Could you check a few things on this model? Use its own coordinates, in mm. Face numbers are marked on the shaded views. A direction names the side the tool comes from. Give positions to 0.01 mm unless a question says otherwise; leave off trailing zeros. Order: outer loops, then holes, each group sorted by start corner. A loop starts at its lowest first (then second) coordinate and runs counter-clockwise, first axis right, second up. Notation, with made-up numbers: M -19,42 L -12,42 A27 cw -12,69 Z; hole C -4,12.5 d7. An arc over 180 degrees is marked long. Answer in a Markdown table with one row per item. Add a question column.
```python
from build123d import *

# Parameters (mm, degrees)
SKETCH1_R                = 21
BOSS_EXTRUDE1_DEPTH      = 35
BOSS_EXTRUDE2_DEPTH      = 100
BOSS_EXTRUDE2_DEPTH_BACK = 18
CUT_EXTRUDE2_DEPTH       = 15
SKETCH7_W                = 9
SKETCH7_H                = 30
CUT_EXTRUDE3_DEPTH       = 7
SKETCH8_R                = 1.55
CUT_EXTRUDE4_DEPTH       = 7
SKETCH9_R                = 16.75
CUT_EXTRUDE5_DEPTH       = 20
CUT_EXTRUDE6_DEPTH       = 20
SKETCH11_R               = 1.65
CUT_EXTRUDE9_DEPTH       = 25
SKETCH12_R               = 16.75
CUT_EXTRUDE8_DEPTH       = 10
CUT_EXTRUDE8_DEPTH_BACK  = 25
CUT_EXTRUDE10_DEPTH      = 20
SKETCH15_W               = 65
SKETCH15_H               = 20
BOSS_EXTRUDE3_DEPTH      = 24
SKETCH16_W               = 13
SKETCH16_H               = 16
CUT_EXTRUDE11_DEPTH      = 65


with BuildPart() as part:
    # Sketch1 → Boss-Extrude1 (new body)
    with BuildSketch(Plane(origin=(0, 0, 0), x_dir=(0, 0, -1), z_dir=(1, 0, 0))):
        Circle(SKETCH1_R)
    extrude(amount=BOSS_EXTRUDE1_DEPTH)

    # Sketch4 → Boss-Extrude2 (add, two sides)
    with BuildSketch(Plane.XY) as boss_extrude2_sk:
        with BuildLine():
            Line((35, 21), (35, -21))
            ThreePointArc((35, -21), (56, 0), (35, 21))
        make_face()
    extrude(amount=BOSS_EXTRUDE2_DEPTH)
    extrude(boss_extrude2_sk.sketch, amount=-BOSS_EXTRUDE2_DEPTH_BACK)

    # Sketch5 → Cut-Extrude2 (cut)
    with BuildSketch(Plane.XY.offset(100)):
        with BuildLine():
            Line((45, -18.466185313), (45, 18.466185313))
            ThreePointArc((45, 18.466185313), (56, 0), (45, -18.466185313))
        make_face()
    extrude(amount=-CUT_EXTRUDE2_DEPTH, mode=Mode.SUBTRACT)

    # Sketch7 → Cut-Extrude3 (cut)
    with BuildSketch(Plane.ZY.offset(-35)):
        with Locations((92.5, 0)):
            Rectangle(SKETCH7_W, SKETCH7_H)
    extrude(amount=-CUT_EXTRUDE3_DEPTH, mode=Mode.SUBTRACT)

    # Sketch8 → Cut-Extrude4 (cut)
    with BuildSketch(Plane.ZY.offset(-42)):
        with Locations((92.5, 6.5)):
            Circle(SKETCH8_R)
        with Locations((92.5, 0)):
            Circle(SKETCH8_R)
        with Locations((92.5, -6.5)):
            Circle(SKETCH8_R)
    extrude(amount=-CUT_EXTRUDE4_DEPTH, mode=Mode.SUBTRACT)

    # Sketch9 → Cut-Extrude5 (cut)
    with BuildSketch(Plane.ZY):
        Circle(SKETCH9_R)
    extrude(amount=-CUT_EXTRUDE5_DEPTH, mode=Mode.SUBTRACT)

    # Sketch10 → Cut-Extrude6 (cut)
    with BuildSketch(Plane.ZY):
        with BuildLine():
            Line((15.02133973, 14.675127009), (12.173811363, 11.504817117))
            ThreePointArc((12.173811363, 11.504817117), (16.743318767, -0.473050368), (11.504817117, -12.173811363))
            Line((11.504817117, -12.173811363), (14.675127009, -15.02133973))
            ThreePointArc((14.675127009, -15.02133973), (20.998573008, -0.244809363), (15.02133973, 14.675127009))
        make_face()
    extrude(amount=-CUT_EXTRUDE6_DEPTH, mode=Mode.SUBTRACT)

    # Sketch11 → Cut-Extrude9 (cut)
    with BuildSketch(Plane.ZY.offset(-20)):
        with Locations((-8.485281374, 8.485281374)):
            Circle(SKETCH11_R)
        with Locations((8.485281374, 8.485281374)):
            Circle(SKETCH11_R)
        with Locations((8.485281374, -8.485281374)):
            Circle(SKETCH11_R)
        with Locations((-8.485281374, -8.485281374)):
            Circle(SKETCH11_R)
    extrude(amount=-CUT_EXTRUDE9_DEPTH, mode=Mode.SUBTRACT)

    # Sketch12 → Cut-Extrude8 (cut, two sides)
    with BuildSketch(Plane.ZY.offset(-35)) as cut_extrude8_sk:
        Circle(SKETCH12_R)
    extrude(amount=CUT_EXTRUDE8_DEPTH, mode=Mode.SUBTRACT)
    extrude(cut_extrude8_sk.sketch, amount=-CUT_EXTRUDE8_DEPTH_BACK, mode=Mode.SUBTRACT)

    # Sketch14 → Cut-Extrude10 (cut)
    with BuildSketch(Plane.ZY):
        with BuildLine():
            Line((-14.710965935, 14.986243067), (-11.829145313, 11.858913153))
            ThreePointArc((-11.829145313, 11.858913153), (-16.749986774, 0.021049042), (-11.858913153, -11.829145313))
            Line((-11.858913153, -11.829145313), (-14.986243067, -14.710965935))
            ThreePointArc((-14.986243067, -14.710965935), (-20.999097868, 0.194650327), (-14.710965935, 14.986243067))
        make_face()
    extrude(amount=-CUT_EXTRUDE10_DEPTH, mode=Mode.SUBTRACT)

    # Sketch15 → Boss-Extrude3 (add)
    with BuildSketch(Plane.ZY.offset(-35)):
        with Locations((52.5, 0)):
            Rectangle(SKETCH15_W, SKETCH15_H)
    extrude(amount=BOSS_EXTRUDE3_DEPTH)

    # Sketch16 → Cut-Extrude11 (cut)
    with BuildSketch(Plane.XY.offset(85)):
        with Locations((20.5, 0)):
            Rectangle(SKETCH16_W, SKETCH16_H)
    extrude(amount=-CUT_EXTRUDE11_DEPTH, mode=Mode.SUBTRACT)


solid = part.part
```
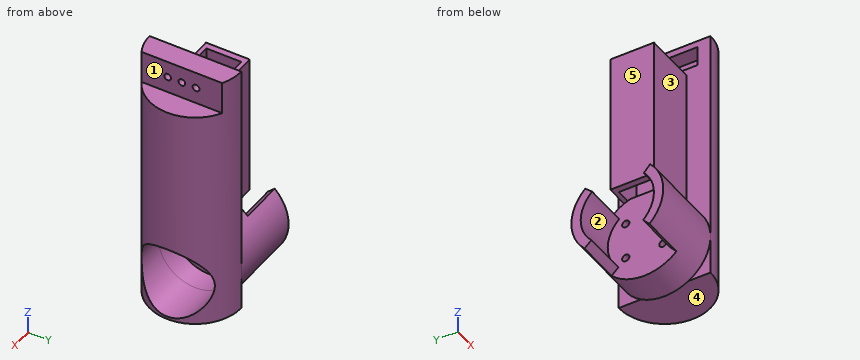
1. Suppose I cut it at D-D on x = 18.5. List the corners of the cut face in (y, z) for me.
2. If I drill on line 1 along Y through (x, z) = (31, 0); line 2 along X through (y, z) = (1, 57); line 3 along Z through (x, y) = (37.5, -4.5), over which ranges is the centre line in solid material (lowest first)? Write a range as [from, to].
3. Suppose I cut it at A-A on z = 92.5. List the corners of the cut face in (x, y) for me.
4. For the marked faces 1, 2, 3, 4 and 5, which set-ups out of +Z, -Z, +X, -X, +Y, -Y let a thin tool reach every point of the face, with its end or its side?
5. Will these pins go through, and if not, where does the flat tip stop? P1, Ø21, axis at y = 4.5, z = 36, coming from the -X side; P2, Ø3, axis at x = 49, z = -5, coming from the -Y side; P3, Ø5, axis at y = 13.5, z = 1.5, coming from the -X side; P4, Ø2.5, axis at y = 0, z = 92.5, coming from the +X side.
6. Suppose I cut it at B-B on y = 0. List the corners of the cut face in (x, z) for me, plus the area to 3 significant figures.
7. Suppose I cut it at C-C on x = 5. List the corners of the cut face in (y, z) for me, plus the area to 3 significant figures.
Findings below:
| question | item | result |
|---|---|---|
| 1 | outline | M -15.02,14.68 A21 ccw -14.71,-14.99 L -11.83,-11.86 A16.75 cw -12.17,11.5 Z; M -10,20 L -8,20 L -8,85 L -10,85 Z; M 8,20 L 10,20 L 10,85 L 8,85 Z; M 11.5,12.17 A16.75 cw 11.86,-11.83 L 14.99,-14.71 A21 ccw 14.68,15.02 Z |
| 2 | line 1 | [-21, -16.75], [16.75, 21] |
| 2 | line 2 | [11, 14], [27, 55.98] |
| 2 | line 3 | [-18, -16.13], [16.13, 88], [97, 100] |
| 3 | outline | M 35,-21 A21 ccw 45,-18.47 L 45,-8.05 L 42,-8.05 L 42,-15 L 35,-15 Z; M 35,15 L 42,15 L 42,8.05 L 45,8.05 L 45,18.47 A21 ccw 35,21 Z; M 42,-4.95 L 45,-4.95 L 45,-1.55 L 42,-1.55 Z; M 42,1.55 L 45,1.55 L 45,4.95 L 42,4.95 Z |
| 4 | face 1 | +Z, +X, +Y, -Y |
| 4 | face 2 | -X |
| 4 | face 3 | +Z, -X, -Y |
| 4 | face 4 | -Z, +X, +Y, -Y |
| 4 | face 5 | +Z, -Z, -X, +Y, -Y |
| 5 | P1 | x = 11 |
| 5 | P2 | y = -16.87 |
| 5 | P3 | x = 20 |
| 5 | P4 | through |
| 6 | outline | M 11,20 L 14,20 L 14,85 L 11,85 Z; M 20,-21 L 35,-21 L 35,-18 L 56,-18 L 56,-16.75 L 25,-16.75 L 25,16.75 L 56,16.75 L 56,85 L 45,85 L 45,90.95 L 42,90.95 L 42,88 L 35,88 L 35,85 L 27,85 L 27,20 L 20,20 Z; M 35,97 L 42,97 L 42,94.05 L 45,94.05 L 45,100 L 35,100 Z |
| 6 | area | 2,530 mm2 |
| 7 | outline | M -15.02,14.68 A21 ccw -14.71,-14.99 L -11.83,-11.86 A16.75 cw -12.17,11.5 Z; M 11.5,12.17 A16.75 cw 11.86,-11.83 L 14.99,-14.71 A21 ccw 14.68,15.02 Z |
| 7 | area | 252 mm2 |
